from build123d import *

# Parameters (mm, degrees)
CORTAR_EXTRUIR1_DEPTH      = 7
CROQUIS3_R                 = 1
CORTAR_EXTRUIR2_DEPTH      = 7
CROQUIS4_R                 = 1.855
CROQUIS4_R_2               = 1.435
CORTAR_EXTRUIR3_DEPTH      = 28
CROQUIS5_R                 = 1.435
CORTAR_EXTRUIR4_DEPTH      = 10.0000001
CORTAR_EXTRUIR4_DEPTH_BACK = 10.0000001


with BuildPart() as part:
    # Croquis1 → Revolución1 (revolve)
    with BuildSketch(Plane(origin=(0, 0, 0), x_dir=(1, 0, 0), z_dir=(0, 1, 0))):
        Polygon((10, 0), (10, 6), (25, 6), (25, 9), (7, 9), (7, 6), (0, 6), (0, 0), align=None)
    revolve(axis=Axis((-57.080066138, 0, 0), (1, 0, 0)))

    # Croquis2 → Cortar-Extruir1 (cut)
    with BuildSketch(Plane.ZY):
        with BuildLine():
            Line((-1, 1.5), (1, 1.5))
            ThreePointArc((1, 1.5), (2.5, 0), (1, -1.5))
            Line((1, -1.5), (-1, -1.5))
            ThreePointArc((-1, -1.5), (-2.5, 0), (-1, 1.5))
        make_face()
    extrude(amount=-CORTAR_EXTRUIR1_DEPTH, mode=Mode.SUBTRACT)

    # Croquis3 → Cortar-Extruir2 (cut, symmetric)
    with BuildSketch(Plane(origin=(0, 0, 0), x_dir=(1, 0, 0), z_dir=(0, 1, 0))):
        with Locations((3.5, 0)):
            Circle(CROQUIS3_R)
    extrude(amount=CORTAR_EXTRUIR2_DEPTH, both=True, mode=Mode.SUBTRACT)

    # Croquis4 → Cortar-Extruir3 (cut)
    with BuildSketch(Plane(origin=(0, -9, 0), x_dir=(-1, 0, 0), z_dir=(0, -1, 0))):
        with Locations((-15.195, 0)):
            Circle(CROQUIS4_R)
        with Locations((-20.055, 0)):
            Circle(CROQUIS4_R_2)
    extrude(amount=-CORTAR_EXTRUIR3_DEPTH, mode=Mode.SUBTRACT)

    # Croquis5 → Cortar-Extruir4 (cut, two sides)
    with BuildSketch(Plane.XY) as cortar_extruir4_sk:
        with Locations((17.6, 0)):
            Circle(CROQUIS5_R)
    extrude(amount=CORTAR_EXTRUIR4_DEPTH, mode=Mode.SUBTRACT)
    extrude(cortar_extruir4_sk.sketch, amount=-CORTAR_EXTRUIR4_DEPTH_BACK, mode=Mode.SUBTRACT)


solid = part.part
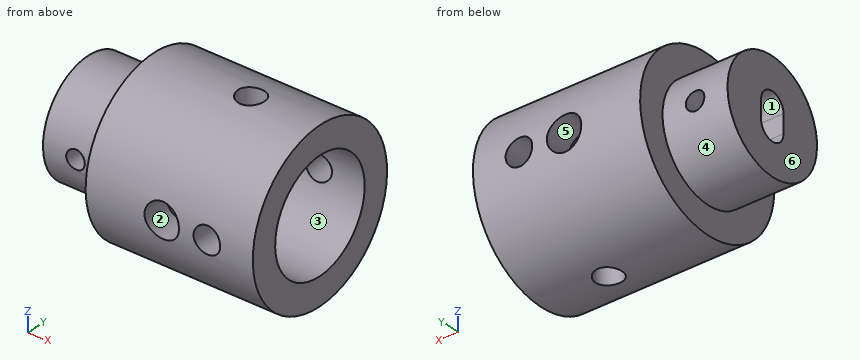
Read the model definition and answer for the solid it produces. Units are mm, in the model's axes. Face numbers are marked on the shaded views. A direction names the side the tool comes from. Round coordinates to 2 decimals unless told otherwise and drop trailing zeros. Order: outer loops, then holes, each group sorted by start corner. A loop starts at its lowest first (then second) coordinate and runs counter-clockwise, first axis right, second up. Notation, with made-up numbers: (-2, 15.25) - (35, 15.25) arc R31 ccw to (35, 48.25) - close; hole circle Ø1 at (-9.5, -27). An arc over 180 degrees is marked (long way). Use one line per item in the form item = value. Start each with the question number.
(1) The part is cut by section A-A (y = 0). Give the vertices of the cut face in (x, z) (3 decimals), then the cut area to 3 significant figures.
(2) The part is cut by section C-C (z = 6.75). Give the vertices of the cut face in (x, y) (3 decimals), then the cut area to 3 significant figures.
(3) Find the intervals of material crossed by line 1 along X through (y, z) = (7.1, 0); line 2 along X through (y, z) = (0, -7.05) (3 decimals); line 3 along X through (y, z) = (-5, -7.25), in increasing order. Write a range as from..to.
(4) Determine the mould class of the marked faces 4, 5 and 6 for opening direction Z: +Z half, -Z half, draft (parallel to the pull), parting line (faces both ways), or undercut.
(5) Flat-ended cylindrical pins translate along their axes: pin 1 Ø3.5 at (x, z) = (20.055, 0) entering from -Y; pin 2 Ø1 at (x, z) = (6, 0.5) entering from +Y; pin 3 Ø2 at (x, z) = (12, 6) entering from +Y; pin 4 Ø0.6 at (x, z) = (2.5, 0) entering from -Y. Find the tip coordinate at first contact, or state that the pin passes through.
(6) For the marked faces 1, 2 and 3, determine the directions among +Z, -Z, +X, -X, +Y, -Y from which every point of the face is accessible in a straight line to the end or side of a thin tool.
(7) The part is cut by section B-B (x = 17.6). Give the vertices of the cut face in (y, z) (3 decimals), then the cut area to 3 significant figures.
(8) The part is cut by section D-D (y = 6.75). Give the vertices of the cut face in (x, z) (3 decimals), then the cut area to 3 significant figures.
Checked values:
q1.outline = (0, -6) - (7, -6) - (7, -9) - (16.165, -9) - (16.165, -6) - (10, -6) - (10, 6) - (16.165, 6) - (16.165, 9) - (7, 9) - (7, 6) - (0, 6) - (0, 2.5) - (7, 2.5) - (7, -2.5) - (0, -2.5) - close; (19.035, -9) - (25, -9) - (25, -6) - (19.035, -6) - close; (19.035, 6) - (25, 6) - (25, 9) - (19.035, 9) - close
q1.area = 176 mm^2
q2.outline = (7, -5.953) - (25, -5.953) - (25, 5.953) - (7, 5.953) - close; hole circle Ø2.87 at (17.6, 0)
q2.area = 208 mm^2
q3.line_1 = 7..13.34, 17.05..18.62, 21.49..25
q3.line_2 = 7..16.165, 19.035..25
q3.line_3 = 7..25
q4.face_4 = parting line
q4.face_5 = undercut
q4.face_6 = draft
q5.pin_1 = -9
q5.pin_2 = 6
q5.pin_3 = 7.48
q5.pin_4 = -6
q6.face_1 = -X
q6.face_2 = +Y, -Y
q6.face_3 = +X
q7.outline = (-1.435, -8.885) - (-1.435, -5.826) arc R6 cw to (-1.435, 5.826) - (-1.435, 8.885) arc R9 ccw to start; (1.435, -8.885) arc R9 ccw to (1.435, 8.885) - (1.435, 5.826) arc R6 cw to (1.435, -5.826) - close
q7.area = 124 mm^2
q8.outline = (7, -5.953) - (25, -5.953) - (25, 5.953) - (7, 5.953) - close; hole circle Ø3.71 at (15.195, 0); hole circle Ø2.87 at (20.055, 0)
q8.area = 197 mm^2
